from build123d import *

# Parameters (mm, degrees)
BOX018_W         = 2
BOX018_H         = 2
BOX018_DEPTH     = 15
ARRAY003_X_COUNT = 2
ARRAY003_X_PITCH = 15
ARRAY003_Y_COUNT = 2
ARRAY003_Y_PITCH = 13
BOX017_W         = 25
BOX017_H         = 20
BOX017_DEPTH     = 25
BOX016_W         = 17
BOX016_H         = 15
BOX016_DEPTH     = 22


with BuildPart() as obj1:
    # Box018 → Box018 (new body)
    with BuildSketch(Plane.XY):
        with Locations((1, 1)):
            Rectangle(BOX018_W, BOX018_H)
    extrude(amount=BOX018_DEPTH)

    # Array003 X: obj1_2


with BuildPart() as obj1_1:
    add(obj1.part)
    with Locations(*[(i * ARRAY003_X_PITCH, 0, 0) for i in range(1, ARRAY003_X_COUNT)]):
        add(obj1.part)

    # Array003 Y: obj1_2


with BuildPart() as obj1_2:
    add(obj1_1.part)
    with Locations(*[(0, i * ARRAY003_Y_PITCH, 0) for i in range(1, ARRAY003_Y_COUNT)]):
        add(obj1_1.part)


with BuildPart() as obj2:
    # Box017 → Box017 (new body)
    with BuildSketch(Plane(origin=(2, -2, 2), x_dir=(1, 0, 0), z_dir=(0, 0, 1))):
        with Locations((12.5, 10)):
            Rectangle(BOX017_W, BOX017_H)
    extrude(amount=BOX017_DEPTH)


with BuildPart() as obj3:
    # Box016 → Box016 (new body)
    with BuildSketch(Plane.XY):
        with Locations((8.5, 7.5)):
            Rectangle(BOX016_W, BOX016_H)
    extrude(amount=BOX016_DEPTH)

    # Cut003: cut obj2
    add(obj2.part, mode=Mode.SUBTRACT)


with BuildPart() as obj3_1:
    # Cut003 placement: moved
    add(obj3.part.moved(Location((0, 0, 15))))

    # Fusion005: union obj1
    add(obj1_2.part)


solid = obj3_1.part
Can you work these out from the model? Positions are in its coordinate system, mm. A direction names the side the tool comes from. Round coordinates to 2 decimals unless told otherwise and drop trailing zeros. Write each loop counter-clockwise with the first axis right and the second up, starting at its lowest first coordinate (ties: lowest second). Pieces come first, ordered by that corner, then holes. Notation, with made-up numbers: M 8.25,57.25 L 44.25,57.25 A28 cw 44.25,89.25 Z; hole C -31.75,-5.5 d9. An arc over 180 degrees is marked long. Use a Markdown table: item, result.
Item 1: We'd pull the mould along X, two halves only. Please class faces 4 (the face through (17, 7.5, 15.4)), 5 (the face through (2, 1, 7)), 6 (the face through (0, 7, 22)), 7 (the face through (16, 2, 7)): released by +X, released by -X, zero draft, split by the parting line, or undercut.
Found:
| item | result |
|---|---|
| face 4 | released by +X |
| face 5 | undercut |
| face 6 | released by -X |
| face 7 | zero draft |
Item 2: I want a section at A-A (z = 5.5). List the corners of the cut face in (x, y) for me.
Found:
| item | result |
|---|---|
| outline | M 0,0 L 2,0 L 2,2 L 0,2 Z; M 0,13 L 2,13 L 2,15 L 0,15 Z; M 15,0 L 17,0 L 17,2 L 15,2 Z; M 15,13 L 17,13 L 17,15 L 15,15 Z |
Item 3: For pin 1 Ø4.5 at (y, z) = (7, 27) entering from +X; pin 2 Ø8 at (x, y) = (7.5, 2) entering from +Z; pin 3 Ø7.5 at (x, y) = (6, 7.5) entering from -Z, each with a flat end and sliding along its axis, tell me the tip position at first contact or that it passes through.
Found:
| item | result |
|---|---|
| pin 1 | stops at x = 2 |
| pin 2 | stops at z = 17 |
| pin 3 | stops at z = 15 |
Item 4: I want a section at C-C (x = 1.5). List the corners of the cut face in (y, z) for me, and give its area (3 significant figures).
Found:
| item | result |
|---|---|
| outline | M 0,0 L 2,0 L 2,15 L 13,15 L 13,0 L 15,0 L 15,37 L 0,37 Z |
| area | 390 mm2 |
Item 5: Which directions (+Z, -Z, +X, -X, +Y, -Y) give clear straight access to the entire face, cutting with the end or side of a thin tool? Please do faces 1 (the face through (9, 8, 17)), 2 (the face through (15, 1, 7)), 3 (the face through (1, 2, 7)).
Found:
| item | result |
|---|---|
| face 1 | +Z, +X, +Y, -Y |
| face 2 | -Z, +Y, -Y |
| face 3 | -Z, +X, -X |
Item 6: If I drill on line 1 along Z through (x, y) = (16, 11.75); line 2 along Z through (x, y) = (1, 7.75); line 3 along X through (y, z) = (14, 17.5), over which ranges is the centre line in solid material (lowest first)? Write a range as [from, to].
Found:
| item | result |
|---|---|
| line 1 | z = [15, 17] |
| line 2 | z = [15, 37] |
| line 3 | x = [0, 2] |
Item 7: I want a section at B-B (y = 13.5). List the corners of the cut face in (x, z) for me.
Found:
| item | result |
|---|---|
| outline | M 0,0 L 2,0 L 2,15 L 15,15 L 15,0 L 17,0 L 17,17 L 2,17 L 2,37 L 0,37 Z |
Item 8: I want a section at D-D (z = 29.5). List the corners of the cut face in (x, y) for me, and give its area (3 significant figures).
Found:
| item | result |
|---|---|
| outline | M 0,0 L 2,0 L 2,15 L 0,15 Z |
| area | 30.0 mm2 |
